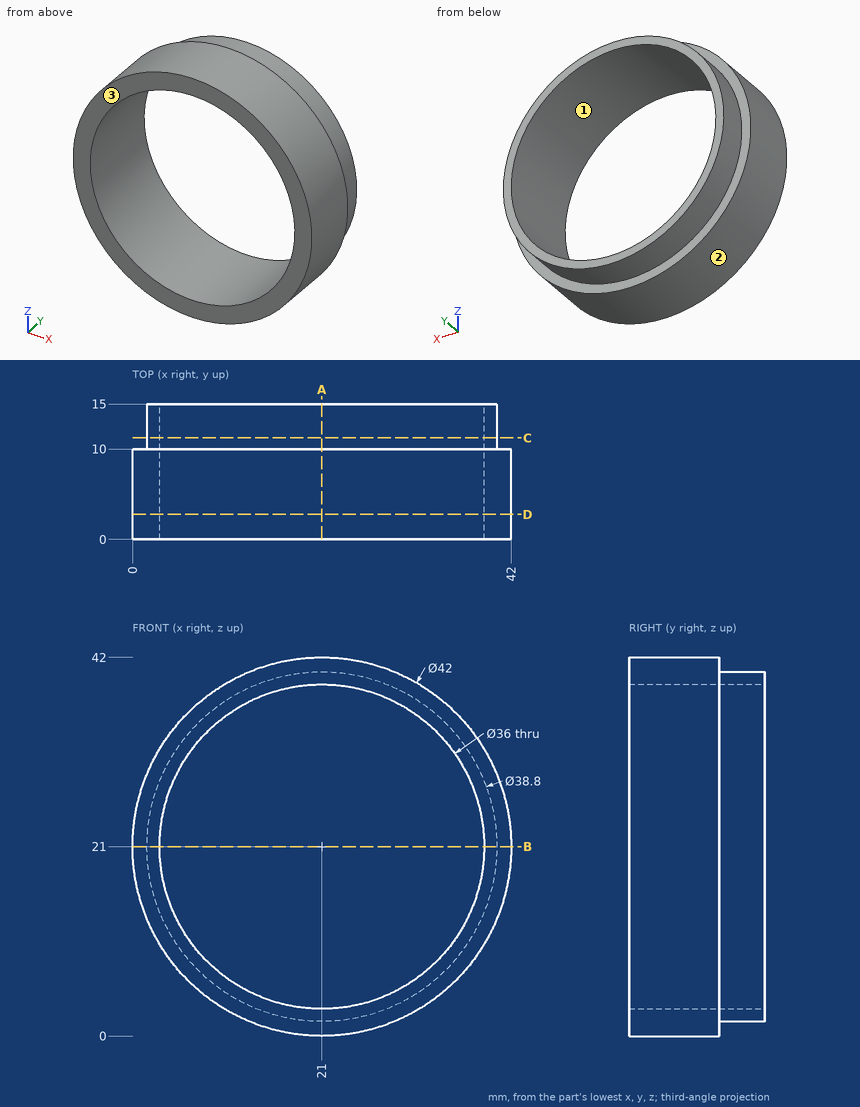
Study the drawing (mm; zero at the part's minimum x, y, z) and answer. Round coordinates to 2 decimals unless told otherwise and drop trailing zeros. Write each loop counter-clockwise with the first axis right and the second up, starting at its lowest first coordinate (ties: lowest second). Pieces come first, ordered by that corner, then holes.
1) A cutting plane is placed at B-B on z = 21. Determine the outline of the cut face in (x, y).
2) Consider probe 1 along X at (y, z) = (9.25, 21); probe 2 along X at (y, z) = (13, 20.5); probe 3 along Y at (x, z) = (35, 7). Determine where each line is inside the solid, lowest interval first.
3) A cutting plane is placed at A-A on x = 21. Determine the outline of the cut face in (y, z).
4) A cutting plane is placed at D-D on y = 2.75. Determine the outline of the cut face in (x, z).
5) Flat-ended cylindrical pins translate along their axes: P1, Ø2, axis at x = 12, y = 13.5, coming from the +Z side; P2, Ø1, axis at x = 7.5, z = 31, coming from the -Y side; P3, Ø5, axis at y = 6, z = 17.5, coming from the -X side; P4, Ø6, axis at y = 9, z = 30.5, coming from the -X side. Find the tip coordinate at first contact, or state that the pin passes through.
6) Determine the mould class of the marked faces 1, 2 and 3 for opening direction X: pulls with the +X half, pulls with the -X half, needs draft (parallel to the pull), parting line crosses it, or undercut.
7) A cutting plane is placed at C-C on y = 11.25. Determine the outline of the cut face in (x, z), and give its area (3 significant figures).
Entries:
1. outline: (0, 0) - (3, 0) - (3, 15) - (1.6, 15) - (1.6, 10) - (0, 10) - close; (39, 0) - (42, 0) - (42, 10) - (40.4, 10) - (40.4, 15) - (39, 15) - close
2. probe 1: x = 0 to 3, 39 to 42
2. probe 2: x = 1.61 to 3.01, 38.99 to 40.39
2. probe 3: y = 0 to 10
3. outline: (0, 0) - (10, 0) - (10, 1.6) - (15, 1.6) - (15, 3) - (0, 3) - close; (0, 39) - (15, 39) - (15, 40.4) - (10, 40.4) - (10, 42) - (0, 42) - close
4. outline: circle Ø42 at (21, 21); hole circle Ø36 at (21, 21)
5. P1: stops at z = 38.67
5. P2: passes through
5. P3: stops at x = 0.02
5. P4: stops at x = 1.03
6. face 1: undercut
6. face 2: parting line crosses it
6. face 3: needs draft
7. outline: circle Ø38.8 at (21, 21); hole circle Ø36 at (21, 21)
7. area: 164 mm2
